Input: part model. Units: mm. Frame: model coordinates. A direction names the side the tool comes from. Coordinates: 2 decimals unless noted, no trailing zeros. Order: outer loops, then holes, each group sorted by start corner. A loop starts at its lowest first (then second) coordinate and runs counter-clockwise, first axis right, second up. Notation, with made-up numbers: M 4.5,39 L 13.5,39 A31 cw 13.5,71 Z; hole C -17,-26 d11. An arc over 180 degrees is marked long. Answer in a Markdown table with one row per item.
from build123d import *

# Parameters (mm, degrees)
F0_W     = 5.113421
F0_H     = 6.01579
F1_DEPTH = 200


with BuildPart() as f1:
    # F0 (on Right) → F1 (new body)
    with BuildSketch(Plane.YZ):
        with Locations((-2.55671, -23.16079)):
            Rectangle(F0_W, F0_H)
        Polygon((-59.857104, -30.078948), (0, -30.078948), (0, -26.168685), (-5.113421, -26.168685), (-55.646054, -26.168685), (-55.646054, 43.313686), (-26.168685, 43.313686), (-26.168685, 48.126314), (-59.857104, 48.126314), align=None)
    extrude(amount=F1_DEPTH)


solid = f1.part
1) Mould query, pull axis Y, two halves, no side actions, for faces 1 (the face through (99, 0, -28)), 2 (the face through (99, -5.113, -23)), 3 (the face through (0, -57, 9)). Classes: +Y half, -Y half, draft (parallel to the pull), parting line (faces both ways), or undercut.
Resolved:
| item | result |
|---|---|
| face 1 | +Y half |
| face 2 | undercut |
| face 3 | draft |
2) Reachability of faces 4 (the face through (99, -41, 43.314)), 5 (the face through (99, -30, -26.169)), 6 (the face through (99, -26.169, 46)) from +Z, -Z, +X, -X, +Y, -Y: full face, straight path, thin tool, end or side. Return the list, or none.
Resolved:
| item | result |
|---|---|
| face 4 | +X, -X, +Y |
| face 5 | +X, -X |
| face 6 | +Z, +X, -X, +Y |
3) Cut plane B-B, the plane x = 152.5. Output: boundary loops of the cut face in (y, z), and give its area (3 significant figures).
Resolved:
| item | result |
|---|---|
| outline | M -59.86,-30.08 L 0,-30.08 L 0,-20.15 L -5.11,-20.15 L -5.11,-26.17 L -55.65,-26.17 L -55.65,43.31 L -26.17,43.31 L -26.17,48.13 L -59.86,48.13 Z |
| area | 720 mm2 |
4) Material intervals for probe 1 along Z at (x, y) = (188, -30); probe 2 along Z at (x, y) = (151, -17); probe 3 along Y at (x, z) = (189.5, 35), sorted ascending.
Resolved:
| item | result |
|---|---|
| probe 1 | z = -30.08 to -26.17, 43.31 to 48.13 |
| probe 2 | z = -30.08 to -26.17 |
| probe 3 | y = -59.86 to -55.65 |
5) Cut plane D-D, the plane y = -7. Output: boundary loops of the cut face in (x, z), and give its area (3 significant figures).
Resolved:
| item | result |
|---|---|
| outline | M 0,-30.08 L 200,-30.08 L 200,-26.17 L 0,-26.17 Z |
| area | 782 mm2 |
6) Cut plane A-A, the plane y = -35. Output: boundary loops of the cut face in (x, z).
Resolved:
| item | result |
|---|---|
| outline | M 0,-30.08 L 200,-30.08 L 200,-26.17 L 0,-26.17 Z; M 0,43.31 L 200,43.31 L 200,48.13 L 0,48.13 Z |
7) Cut plane C-C, the plane z = 41. Output: boundary loops of the cut face in (x, y), and give its area (3 significant figures).
Resolved:
| item | result |
|---|---|
| outline | M 0,-59.86 L 200,-59.86 L 200,-55.65 L 0,-55.65 Z |
| area | 842 mm2 |
8) Contact query for flat-ended pins moving along their axis: pin 1 (2.5 mm diameter, centred on x = 88, z = 45, fed in from +Y); pin 2 (3 mm diameter, centred on x = 153.5, y = -7, fed in from +Z); pin 3 (1 mm diameter, centred on x = 87, z = 7.5, fed in from +Y). Output: stop coordinate, or through.
Resolved:
| item | result |
|---|---|
| pin 1 | stops at y = -26.17 |
| pin 2 | stops at z = -26.17 |
| pin 3 | stops at y = -55.65 |
